CAD build for the part. Positions are in the model's coordinates, mm. Face numbers are marked on the shaded views. A direction names the side the tool comes from. Coordinates: 2 decimals unless noted, no trailing zeros. Order: outer loops, then holes, each group sorted by start corner. A loop starts at its lowest first (then second) coordinate and runs counter-clockwise, first axis right, second up. Notation, with made-up numbers: (87, 8.5) -> (134, 8.5) arc R23 cw to (134, 19.5) -> close; hole circle Ø1 at (-22.5, 34). An arc over 180 degrees is marked (long way). Use one line per item in the form item = value. Start each with the question number.
from build123d import *

# Parameters (mm, degrees)
BOSS_EXTRUDE1_DEPTH = 38.1
FILLET1_R           = 2.54
SKETCH2_W           = 3.048
SKETCH2_H           = 2
SKETCH2_W_2         = 6.87382658
SKETCH2_H_2         = 19.05
CUT_EXTRUDE1_DEPTH  = 12.7
SKETCH3_W           = 3
SKETCH3_H           = 25.822446998
BOSS_EXTRUDE2_DEPTH = 6.35
SKETCH4_W           = 3
SKETCH4_H           = 25.822446998
BOSS_EXTRUDE4_DEPTH = 6.35
FILLET3_R           = 42.545
FILLET4_R           = 6.35


# Some blends are built 0.0001 mm under size
with BuildPart() as part:
    # Sketch1 → Boss-Extrude1 (new body)
    with BuildSketch(Plane.XY):
        Polygon((-1.3335, 40.099523747), (-3.3654746, 40.109683747), (-3.566025525, 0), (3.566025525, 0), (3.3654746, 40.109683747), (1.3335, 40.099523747), (1.524, 2), (-1.524, 2), align=None)
        Polygon((-1.3096875, 44.861964215), (-1.3335, 40.099523747), (-3.3654746, 40.109683747), (-3.3416621, 44.872124215), align=None)
    extrude(amount=BOSS_EXTRUDE1_DEPTH)

    # Fillet1
    # the kernel refuses this fillet: 2.54 mm, written as the material it takes off along each edge
    with BuildSketch(Plane(origin=(1.3335, 40.099523747, -6.221703947), x_dir=(0.005000000000000079, -0.999987499921874, 0), z_dir=(0, 0, 1))) as fillet1_piece_1:
        with BuildLine():
            CenterArc((2.488681579, 2.54), FILLET1_R, 191.536959033, 78.463040967)
            Line((0, 2.032), (-0.049773632, 2.02184))
            ThreePointArc((-0.049773632, 2.02184), (-0.0508, 1.016), (-0.0508, 0))
            Line((-0.0508, 0), (0, -0.0508))
            Line((0, -0.0508), (2.488681579, -0.0508))
            Line((2.488681579, -0.0508), (2.488681579, 0))
        make_face()
    extrude(amount=50.543407893, mode=Mode.SUBTRACT)
    with BuildSketch(Plane(origin=(-1.3096875, 44.861964215, -6.221703947), x_dir=(-0.005000000000000297, -0.999987499921874, 0), z_dir=(0, 0, 1))) as fillet1_piece_2:
        with BuildLine():
            CenterArc((2.488681579, -2.54), FILLET1_R, 90, 78.463040967)
            Line((0, -2.032), (-0.049773632, -2.02184))
            ThreePointArc((-0.049773632, -2.02184), (-0.0508, -1.016), (-0.0508, 0))
            Line((-0.0508, 0), (0, 0.0508))
            Line((0, 0.0508), (2.488681579, 0.0508))
            Line((2.488681579, 0.0508), (2.488681579, 0))
        make_face()
    extrude(amount=50.543407893, mode=Mode.SUBTRACT)

    # Sketch2 → Cut-Extrude1 (cut)
    with BuildSketch(Plane.XY.offset(38.1)):
        with Locations((0, 1)):
            Rectangle(SKETCH2_W, SKETCH2_H)
        with Locations((0, 35.347124215)):
            Rectangle(SKETCH2_W_2, SKETCH2_H_2)
    extrude(amount=-CUT_EXTRUDE1_DEPTH, mode=Mode.SUBTRACT)

    # Sketch3 → Boss-Extrude2 (add)
    with BuildSketch(Plane(origin=(3.565936375, 0.017829905, 0), x_dir=(0, 0, -1), z_dir=(0.9999874999218742, 0.004999999999999631, 0))):
        with Locations((-23.9, 12.893393371)):
            Rectangle(SKETCH3_W, SKETCH3_H)
        with Locations((-29.948, 12.893393371)):
            Rectangle(SKETCH3_W, SKETCH3_H)
    extrude(amount=BOSS_EXTRUDE2_DEPTH)

    # Sketch4 → Boss-Extrude4 (add)
    with BuildSketch(Plane(origin=(-3.565936375, 0.017829905, 0), x_dir=(0, 0, 1), z_dir=(-0.9999874999218742, 0.004999999999999631, 0))):
        with Locations((29.948, 12.893393371)):
            Rectangle(SKETCH4_W, SKETCH4_H)
        with Locations((23.9, 12.893393371)):
            Rectangle(SKETCH4_W, SKETCH4_H)
    extrude(amount=BOSS_EXTRUDE4_DEPTH)

    # Fillet3
    # the kernel refuses this fillet: 42.545 mm, written as the material it adds along each edge
    with BuildSketch(Plane(origin=(3.43691329, 25.822124215, 22.4), x_dir=(0, 0, -1), z_dir=(0.004999999999999631, -0.9999874999218742, 0))) as fillet3_piece_1:
        with BuildLine():
            CenterArc((22.360657414, 42.545), FILLET3_R, 238.292930672, 31.707069328)
            Line((0, 6.35), (0, 0))
            Line((0, 0), (22.360657414, 0))
        make_face()
    extrude(amount=25.822446998)
    with BuildSketch(Plane(origin=(-3.43691329, 25.822124215, 22.4), x_dir=(0, 0, -1), z_dir=(-0.004999999999999631, -0.9999874999218742, 0))) as fillet3_piece_2:
        with BuildLine():
            CenterArc((22.360657414, -42.545), FILLET3_R, 90, 31.707069328)
            Line((0, -6.35), (0, 0))
            Line((0, 0), (22.360657414, 0))
        make_face()
    extrude(amount=25.822446998)

    # Fillet4
    fillet4_edges = [part.edges().sort_by_distance(p)[0] for p in [
        (3.501469408, 12.911062108, 31.448),
        (-3.501469408, 12.911062108, 31.448),
    ]]
    fillet(fillet4_edges, radius=FILLET4_R - 0.0001)  # a hair under: the kernel refuses the full size


solid = part.part
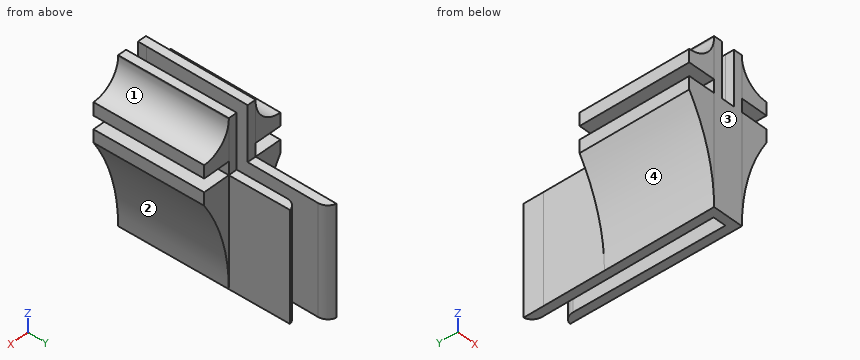
1) Cut at B-B on z = 24. Give the cut face in (x, y), then the cut area to 3 significant figures.
2) Cut at C-C on z = 15. Give the cut face in (x, y).
3) Drop flat-ended pins along their axis: P1, Ø1.9, axis at x = 6, y = 18, coming from the +Z side; P2, Ø1.9, axis at x = -7.5, y = 14, coming from the -Z side; P3, Ø1, axis at y = 25.5, z = 30, coming from the -X side; P4, Ø2, axis at x = -6.5, z = 4, coming from the +Y side. Give the stop position or say it passes through.
4) Cut at A-A on y = 35.5. Give the cut face in (x, z), then the cut area to 3 significant figures.
5) 3-axis set-ups, long thin cutter, end or side, ignore diameter. For the marked faces 1, 2, 3 and 4: which of +Z, -Z, +X, -X, +Y, -Y reach the whole face in a straight line?
6) Probe L1, parallel to X at y = 28.5, z = 24; L2, parallel to Z at x = 1.5, y = 33; L3, parallel to Y at x = -6, z = 31. List the from-to ranges inside material, lowest first.
Values follow:
q1.outline = (-9.92, 0.03) -> (-3.57, 0) -> (3.57, 0) -> (9.92, 0.03) -> (9.79, 25.85) -> (3.44, 25.82) -> (3.37, 40.11) arc R2.54 ccw to (1.35, 37.61) -> (1.52, 2) -> (-1.52, 2) -> (-1.32, 42.37) arc R2.54 ccw to (-3.34, 44.87) -> (-3.44, 25.82) -> (-9.79, 25.85) -> close
q1.area = 504 mm^2
q2.outline = (-6.28, 0.01) -> (-3.57, 0) -> (3.57, 0) -> (6.28, 0.01) -> (6.15, 25.84) -> (3.44, 25.82) -> (3.37, 40.11) arc R2.54 ccw to (1.35, 37.61) -> (1.52, 2) -> (-1.52, 2) -> (-1.32, 42.37) arc R2.54 ccw to (-3.34, 44.87) -> (-3.44, 25.82) -> (-6.15, 25.84) -> close
q3.P1 = 33.61
q3.P2 = 15.87
q3.P3 = -9.79
q3.P4 = through
q4.outline = (-3.39, 0) -> (-1.36, 0) -> (-1.36, 25.4) -> (-3.39, 25.4) -> close; (1.36, 0) -> (3.39, 0) -> (3.39, 25.4) -> (1.36, 25.4) -> close
q4.area = 103 mm^2
q5.face_1 = +Z, +X, +Y
q5.face_2 = -Z, +X, +Y
q5.face_3 = +Z, -Z, +X, -X, -Y
q5.face_4 = -Z, -X, +Y
q6.L1 = -3.42 to -1.39, 1.39 to 3.42
q6.L2 = 0 to 25.4
q6.L3 = 0.01 to 25.83
